Can you work these out from the drawing? Everything is in mm from the part's minimum corner. A direction names the side the tool comes from. Coordinates: 2 decimals unless noted, no trailing zeros. Loops run counter-clockwise (first coordinate to the right, second up) from the corner with the lowest first, then second, coordinate; pieces in that order, holes last. Notation, with made-up numbers: M -23,9.25 L 26,9.25 A36 cw 26,46.25 Z; hole C 38.5,35 d6. An arc over 180 degrees is marked long. Write each question's results on one line, items separated by ' | '.
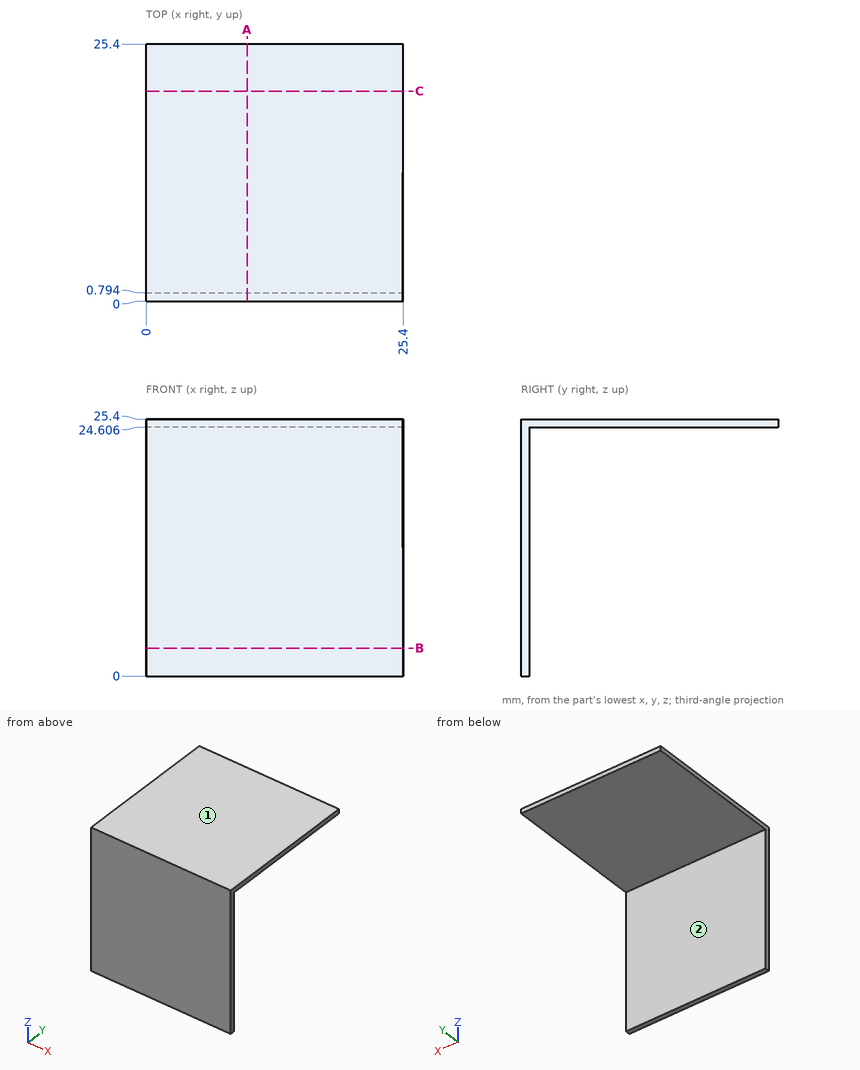
(1) Will these pins go through, and if not, where does the flat tip stop? P1, Ø4, axis at x = 19.5, z = 13, coming from the +Y side; P2, Ø3, axis at x = 11.5, y = 8, coming from the -Z side.
Reported:
P1: stops at y = 0.79 | P2: stops at z = 24.61
(2) Imagine slicing it at C-C, the plane y = 20.75. List the corners of the cut face in (x, z) for me.
Reported:
outline: M 0,24.61 L 25.4,24.61 L 25.4,25.4 L 0,25.4 Z
(3) Imagine slicing it at B-B, the plane z = 2.75. List the corners of the cut face in (x, y) for me.
Reported:
outline: M 0,0 L 25.4,0 L 25.4,0.79 L 0,0.79 Z
(4) Which directions (+Z, -Z, +X, -X, +Y, -Y) give clear straight access to the entire face, cutting with the end or side of a thin tool? Please do the marked faces 1 and 2.
Reported:
face 1: +Z, +X, -X, +Y, -Y | face 2: -Z, +X, -X, +Y
(5) Imagine slicing it at A-A, the plane x = 10. List the corners of the cut face in (y, z) for me.
Reported:
outline: M 0,0 L 0.79,0 L 0.79,24.61 L 25.4,24.61 L 25.4,25.4 L 0,25.4 Z
(6) Please list where these lines run through material, in increasing order: probe 1 along Y at (x, z) = (4, 8); probe 2 along Z at (x, y) = (19.25, 10). Write a range as from..to.
Reported:
probe 1: y = 0..0.79 | probe 2: z = 24.61..25.4
